Part model, mm, in its own coordinate system. Face numbers are marked on the shaded views. A direction names the side the tool comes from. Round coordinates to 2 decimals unless told otherwise and drop trailing zeros. Loops run counter-clockwise (first coordinate to the right, second up) from the corner with the lowest first, then second, coordinate; pieces in that order, holes last. Notation, with made-up numbers: M 73,75 L 88,75 A26 ccw 88,106 Z; hole C 17,5 d8. An arc over 180 degrees is marked long. Answer as CSV lines item,"result". Start each with the question number.
Item 1: Mould opens along Y. For the marked faces 4, 5 and 6 say: pulls with the +Y half, pulls with the -Y half, needs draft (parallel to the pull), parting line crosses it, or undercut.
Item 2: Band-saw the part on A-A (y = 0). Give the cut face in (x, z), and give its area (3 significant figures).
Item 3: Wall check: line 1 (X direction, y = -1, z = 4.75); line 2 (Y direction, x = 19.8, z = 5); line 3 (Y direction, x = 11, z = 4.25). Give the ranges that are in metal, low to high.
Item 4: Band-saw the part on B-B (z = 2.25). Give the cut face in (x, y).
Item 5: Drop flat-ended pins along their axis: pin 1 Ø5 at (x, z) = (-16.5, 5.5) entering from +Y; pin 2 Ø3 at (y, z) = (-7, 7) entering from +X; pin 3 Ø1.2 at (x, z) = (22.5, 5) entering from -Y. Give the stop position or say it passes through.
Item 6: Which spindle directions (+Z, -Z, +X, -X, +Y, -Y) get a long thin tool onto all of the face, cutting with end or side? Do the marked faces 1, 2 and 3. Say none if no direction does.
```python
from build123d import *

# Parameters (mm, degrees)
SKETCH1_R               = 25
BOSS_EXTRUDE1_DEPTH     = 10
CUT_EXTRUDE1_DEPTH      = 37.742346142
CUT_EXTRUDE1_DEPTH_BACK = 37.742346142
CUT_EXTRUDE2_DEPTH      = 3
SKETCH5_R               = 2
CUT_EXTRUDE4_DEPTH      = 13
FILLET1_R               = 1
CUT_EXTRUDE6_DEPTH      = 3
CUT_EXTRUDE6_DEPTH_BACK = 3
SKETCH6_W               = 10
SKETCH6_H               = 10
SKETCH7_W               = 10
SKETCH7_H               = 30
BOSS_EXTRUDE2_DEPTH     = 10
SKETCH8_W               = 10
SKETCH8_H               = 10
BOSS_EXTRUDE3_DEPTH     = 10
SKETCH9_W               = 10
SKETCH9_H               = 10
CUT_EXTRUDE7_DEPTH      = 10


with BuildPart() as part:
    # Sketch1 → Boss-Extrude1 (new body)
    with BuildSketch(Plane.XY):
        Circle(SKETCH1_R)
    extrude(amount=BOSS_EXTRUDE1_DEPTH)

    # Sketch2 → Cut-Extrude1 (cut, two sides: drawn at the far end of the back side and taken through both)
    with BuildSketch(Plane.XY.offset(10).offset(-CUT_EXTRUDE1_DEPTH_BACK)):
        Polygon((5, -5), (15, -5), (15, 5), (5, 5), (5, 15), (-5, 15), (-5, 5), (-15, 5), (-15, -5), (-5, -5), (-5, -15), (5, -15), align=None)
    extrude(amount=CUT_EXTRUDE1_DEPTH + CUT_EXTRUDE1_DEPTH_BACK, mode=Mode.SUBTRACT)

    # Sketch4 → Cut-Extrude2 (cut)
    with BuildSketch(Plane.ZY.offset(-15)):
        Polygon((4.759098318, -4.265594884), (8.57366269, -2.341424419), (8.814564373, 1.924170465), (5.240901682, 4.265594884), (1.42633731, 2.341424419), (1.185435627, -1.924170465), align=None)
    extrude(amount=-CUT_EXTRUDE2_DEPTH, mode=Mode.SUBTRACT)

    # Sketch5 → Cut-Extrude4 (cut)
    with BuildSketch(Plane.ZY.offset(-18)):
        with Locations((5, 0)):
            Circle(SKETCH5_R)
    extrude(amount=-CUT_EXTRUDE4_DEPTH, mode=Mode.SUBTRACT)

    # Fillet1
    fillet1_edges = [part.edges().sort_by_distance(p)[0] for p in [
        (-25, 0, 0),
        (-25, 0, 10),
    ]]
    fillet(fillet1_edges, radius=FILLET1_R)

    # Sketch6 → Cut-Extrude6 (cut, two sides: drawn at the far end of the back side and taken through both)
    with BuildSketch(Plane.YZ.offset(24.999151456).offset(-CUT_EXTRUDE6_DEPTH_BACK)):
        with Locations((0, 5)):
            Rectangle(SKETCH6_W, SKETCH6_H)
    extrude(amount=CUT_EXTRUDE6_DEPTH + CUT_EXTRUDE6_DEPTH_BACK, mode=Mode.SUBTRACT)

    # Sketch7 → Boss-Extrude2 (add)
    with BuildSketch(Plane(origin=(0, 0, 0), x_dir=(-1, 0, 0), z_dir=(0, 0, -1))):
        Rectangle(SKETCH7_W, SKETCH7_H)
    extrude(amount=-BOSS_EXTRUDE2_DEPTH)

    # Sketch8 → Boss-Extrude3 (add)
    with BuildSketch(Plane(origin=(0, 0, 0), x_dir=(-1, 0, 0), z_dir=(0, 0, -1))):
        with Locations((10, 0)):
            Rectangle(SKETCH8_W, SKETCH8_H)
    extrude(amount=-BOSS_EXTRUDE3_DEPTH)

    # Sketch9 → Cut-Extrude7 (cut)
    with BuildSketch(Plane(origin=(0, 0, 0), x_dir=(-1, 0, 0), z_dir=(0, 0, -1))):
        with Locations((15, 0)):
            Rectangle(SKETCH9_W, SKETCH9_H)
    extrude(amount=-CUT_EXTRUDE7_DEPTH, mode=Mode.SUBTRACT)


solid = part.part
```
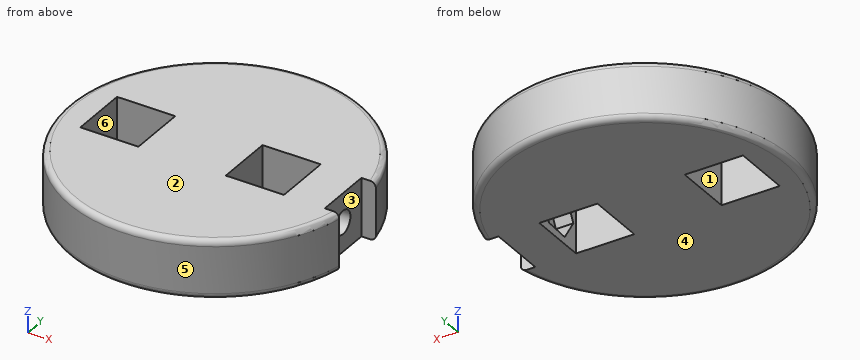
Answer block:
1,face 4,"needs draft"
1,face 5,"parting line crosses it"
1,face 6,"undercut"
2,outline,"M -25,1 A1 ccw -24,0 L -20,0 L -20,10 L -24,10 A1 ccw -25,9 Z; M -10,0 L 5,0 L 5,10 L -10,10 Z; M 15,0 L 22,0 L 22,3 L 18,3 L 18,1.29 L 15,1.29 Z; M 15,8.71 L 18,8.71 L 18,7 L 22,7 L 22,10 L 15,10 Z"
2,area,"231 mm^2"
3,line 1,"x = -24.98 to -20, -10 to 5"
3,line 2,"y = -15.26 to -2, 2 to 15.26"
3,line 3,"y = -22.45 to -5, 5 to 22.45"
4,outline,"M 22,-5 L 22,5 L 24.49,5 A25 ccw long 24.49,-5 Z; hole M -20,-5 L -10,-5 L -10,5 L -20,5 Z; hole M 5,-5 L 15,-5 L 15,-2.62 L 18,-2.62 L 18,2.76 L 15,2.76 L 15,5 L 5,5 Z"
5,pin 1,"stops at y = 20.71"
5,pin 2,"stops at x = 24.39"
5,pin 3,"stops at y = -12.06"
6,face 1,"+Z, -Z"
6,face 2,"+Z, +X, -X, +Y, -Y"
6,face 3,"+Z, -Z, +X"
